Design review of the part built by this model. Coordinates are the model's own, in mm. A direction names the side the tool comes from. Coordinates: 2 decimals unless noted, no trailing zeros. Write each loop counter-clockwise with the first axis right and the second up, starting at its lowest first coordinate (ties: lowest second). Pieces come first, ordered by that corner, then holes.
Q1. For faces 4 (the flat face through (-109, 51.033, 25)), 5 (the flat face through (-57.524, -5, 25)), 6 (the flat face through (-48, 1, 39.652)), 7 (the flat face through (-37.827, -5, 25)), 8 (the flat face through (-99.156, 43, 25)), list the 3-axis set-ups (+Z, -Z, +X, -X, +Y, -Y) from which the entire face can be reached by the end or side of a thin tool; tool diameter is ignored.
Q2. The part is to be moulded in two halves that separate along Y. For faces 1 (the flat face through (-48, 1, 8.861)), 2 (the flat face through (-68, 34.917, 25)), 3 (the flat face through (-48, -30.441, 25)), say which applies: released by +Y, released by -Y, zero draft, split by the parting line, or undercut.
Q3. Take a section at B-B, the plane z = 14.5. Write out the cut boundary in (x, y).
Q4. Take a section at A-A, the plane y = -1. Write out the cut boundary in (x, z).
Q5. For L1, parallel to Y at x = -46.5, z = 26; L2, parallel to Z at x = -43, y = -3; L3, parallel to Y at x = -88, z = 13, list the stretches that pass through material, from the lowest coordinate up.
Q6. Take a section at C-C, the plane x = -43. Write out the cut boundary in (y, z).
Q7. Take a section at D-D, the plane x = -88.5. Write out the cut boundary in (y, z), plus the area to 3 significant figures.
Q8. For pin 1 Ø5 at (y, z) = (39.5, 16.5) entering from +X; pin 2 Ø16 at (x, z) = (-49.5, 19.5) entering from +Y; pin 3 Ø1 at (x, z) = (-61.5, 36) entering from -Y, all flat-tipped, find the tip position at first contact; note any pin that passes through.
from build123d import *

# Parameters (mm, degrees)
F1_DEPTH = 50
F2_W     = 9.416695
F2_H     = 30.791057
F3_DEPTH = 25


with BuildPart() as f1:
    # F0 (on Top) → F1 (new body)
    with BuildSketch(Plane.XY):
        Polygon((-99.156201, 51.032986), (-119.748466, 51.032986), (-119.748466, 19.696943), (-57.524025, 19.696943), (-57.524025, -30.440733), (-37.827082, -30.440733), (-37.827082, 34.917306), (-99.156201, 34.917306), align=None)
    extrude(amount=F1_DEPTH)

    # F2 (on face) → F3 (cut)
    with BuildSketch(Plane.YZ.offset(-37.827082)):
        with Locations((1.276812, 24.256223)):
            Rectangle(F2_W, F2_H)
    extrude(amount=-F3_DEPTH, mode=Mode.SUBTRACT)


solid = f1.part
Responses:
1. face 4: +Z, -Z, +X, -X, +Y
1. face 5: +Z, -Z, -X, -Y
1. face 6: +X, -X
1. face 7: +Z, -Z, +X, +Y, -Y
1. face 8: +Z, -Z, +X, +Y
2. face 1: undercut
2. face 2: released by +Y
2. face 3: released by -Y
3. outline: (-119.75, 19.7) - (-57.52, 19.7) - (-57.52, 5.99) - (-37.83, 5.99) - (-37.83, 34.92) - (-99.16, 34.92) - (-99.16, 51.03) - (-119.75, 51.03) - close; (-57.52, -30.44) - (-37.83, -30.44) - (-37.83, -3.43) - (-57.52, -3.43) - close
4. outline: (-57.52, 0) - (-37.83, 0) - (-37.83, 8.86) - (-57.52, 8.86) - close; (-57.52, 39.65) - (-37.83, 39.65) - (-37.83, 50) - (-57.52, 50) - close
5. L1: y = -30.44 to -3.43, 5.99 to 34.92
5. L2: z = 0 to 8.86, 39.65 to 50
5. L3: y = 19.7 to 34.92
6. outline: (-30.44, 0) - (34.92, 0) - (34.92, 50) - (-30.44, 50) - close; hole (-3.43, 8.86) - (5.99, 8.86) - (5.99, 39.65) - (-3.43, 39.65) - close
7. outline: (19.7, 0) - (34.92, 0) - (34.92, 50) - (19.7, 50) - close
7. area: 761 mm2
8. pin 1: stops at x = -99.16
8. pin 2: stops at y = 34.92
8. pin 3: stops at y = 19.7
